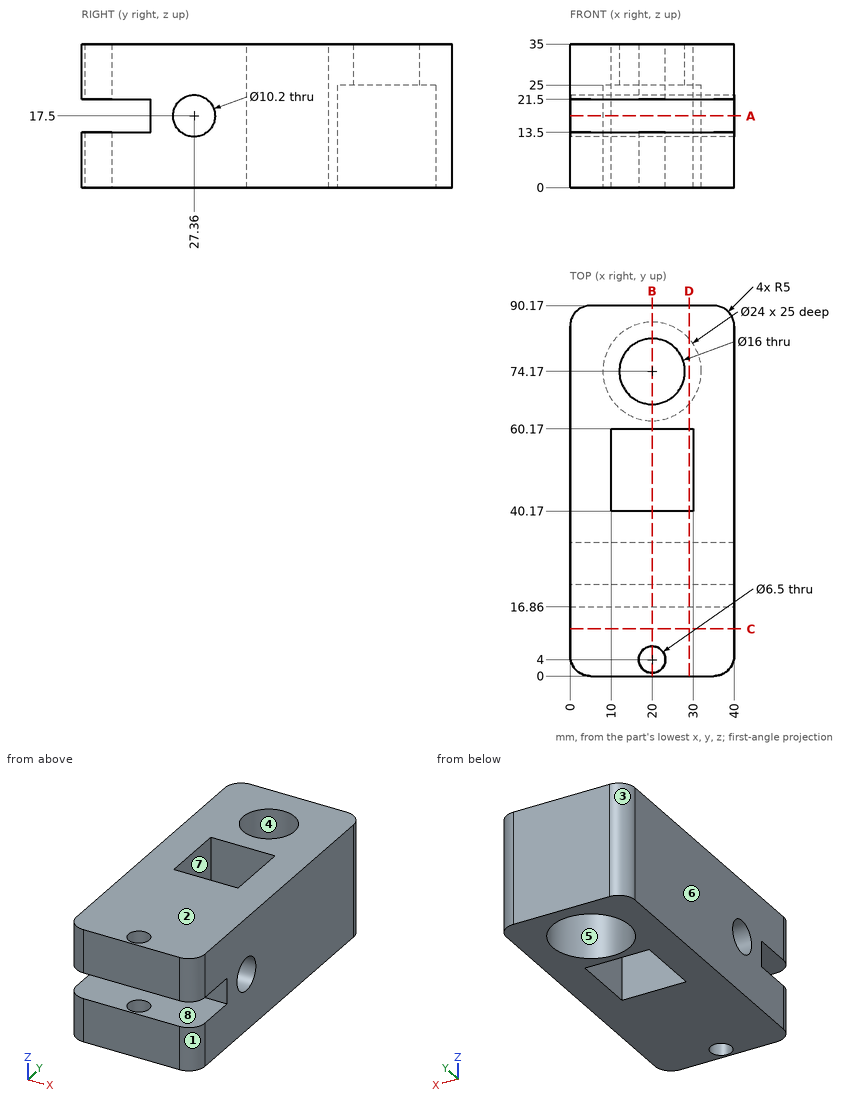
Verification items for this drawing (mm, ordinates from the low corner). A direction names the side the tool comes from. Give positions to 0.01 mm unless a question says otherwise; leave off trailing zeros. Loops run counter-clockwise (first coordinate to the right, second up) from the corner with the lowest first, then second, coordinate; pieces in that order, holes last. Notation, with made-up numbers: M 68.5,7.5 L 113.5,7.5 A23 ccw 113.5,21.5 Z; hole C 4.5,61.5 d9. An arc over 180 degrees is marked long. Answer in a Markdown table with one row per item.
1) Tool access check on the marked faces 5, 6, 7 and 8. Record the directions out of +Z, -Z, +X, -X, +Y, -Y that give a thin tool (end or side, any length) a straight path to the whole face; none if there is none.
Solutions:
| item | result |
|---|---|
| face 5 | -Z |
| face 6 | +Z, -Z, -X, +Y, -Y |
| face 7 | +Z, -Z |
| face 8 | +X, -X, -Y |
2) Cross-section at C-C (y = 11.5). Enter the section's corners in (x, z), plus the area to 3 significant figures.
Solutions:
| item | result |
|---|---|
| outline | M 0,0 L 40,0 L 40,13.5 L 0,13.5 Z; M 0,21.5 L 40,21.5 L 40,35 L 0,35 Z |
| area | 1,080 mm^2 |
3) Cross-section at A-A (z = 17.5). Enter the section's corners in (x, y), plus the area to 3 significant figures.
Solutions:
| item | result |
|---|---|
| outline | M 0,16.86 L 40,16.86 L 40,22.26 L 0,22.26 Z; M 0,32.46 L 40,32.46 L 40,85.17 A5 ccw 35,90.17 L 5,90.17 A5 ccw 0,85.17 Z; hole C 20,74.17 d24; hole M 10,40.17 L 30,40.17 L 30,60.17 L 10,60.17 Z |
| area | 1,660 mm^2 |
4) Mould release check, pull along Y, two halves, no side actions. Record for the marked faces 1, 2, 3 and 4: released by +Y, released by -Y, zero draft, split by the parting line, or undercut.
Solutions:
| item | result |
|---|---|
| face 1 | released by -Y |
| face 2 | zero draft |
| face 3 | released by +Y |
| face 4 | undercut |
5) Cross-section at D-D (x = 29). Enter the section's corners in (y, z).
Solutions:
| item | result |
|---|---|
| outline | M 0,0 L 40.17,0 L 40.17,35 L 0,35 L 0,21.5 L 16.86,21.5 L 16.86,13.5 L 0,13.5 Z; M 60.17,0 L 66.23,0 L 66.23,25 L 82.11,25 L 82.11,0 L 90.17,0 L 90.17,35 L 60.17,35 Z; hole C 27.36,17.5 d10.2 |
6) Cross-section at B-B (x = 20). Count the separate pieces of the cut face and the enclosed holes in it, plus the area to 3 significant figures.
Solutions:
| item | result |
|---|---|
| separate pieces | 5 |
| enclosed holes | 1 |
| area | 1,300 mm^2 |
7) Thickness scan on line 1 (Y direction, x = 20, z = 28.75); line 2 (Z direction, x = 22.5, y = 15); line 3 (Y direction, x = 20, z = 18.5). Record the ranges inside material, lowest first.
Solutions:
| item | result |
|---|---|
| line 1 | y = 0 to 0.75, 7.25 to 40.17, 60.17 to 66.17, 82.17 to 90.17 |
| line 2 | z = 0 to 13.5, 21.5 to 35 |
| line 3 | y = 16.86 to 22.36, 32.36 to 40.17, 60.17 to 62.17, 86.17 to 90.17 |
8) Depth check by flat-ended pin: pin 1 (4 mm diameter, centred on x = 14, z = 19, fed in from -Y). Enter the tip coordinate at first touch or a pass-through.
Solutions:
| item | result |
|---|---|
| pin 1 | stops at y = 16.86 |
